Input: dimensioned drawing with shaded views. Units: mm. Origin: part minimum x, y, z. A direction names the side the tool comes from. Give positions to 0.01 mm unless a question says otherwise; leave off trailing zeros. Order: outer loops, then holes, each group sorted by start corner. A loop starts at its lowest first (then second) coordinate and runs counter-clockwise, first axis right, second up. Notation, with made-up numbers: (87, -7) -> (132, -7) arc R23 cw to (132, 30) -> close; hole circle Ø4 at (13, 62.5). An arc over 180 degrees is marked (long way). One line per question, with ' | ' between items. Start each with the question number.
(1) Section A-A (y = 41.5). Return loops of the section in (x, z), then the cut area to 3 significant figures.
(2) Section D-D (x = 6). Return loops of the section in (y, z).
(3) Set-up query: the marked faces 1 and 2. Return all of +Z, -Z, +X, -X, +Y, -Y with unobstructed straight access to the full face (end or side cutting, diameter ignored); none if empty.
(4) Section C-C (y = 20.5). Return loops of the section in (x, z) (1 decimal).
(5) First-contact query: pin 1 Ø4 at (x, y) = (39.23, 20.5) entering from -Z; pin 2 Ø1.5 at (x, z) = (30, 37) entering from +Y; pin 3 Ø1.5 at (x, y) = (44, 8) entering from -Z. Flat tips, straight axial feed; report the tip coordinate or a pass-through.
(6) Section B-B (x = 34). Return loops of the section in (y, z).
(7) Ray query, L1, parallel to X at y = 27, z = 51; L2, parallel to Z at x = 47, y = 42; L3, parallel to Y at x = 10, z = 3.5. Return the intervals inside material, ascending.
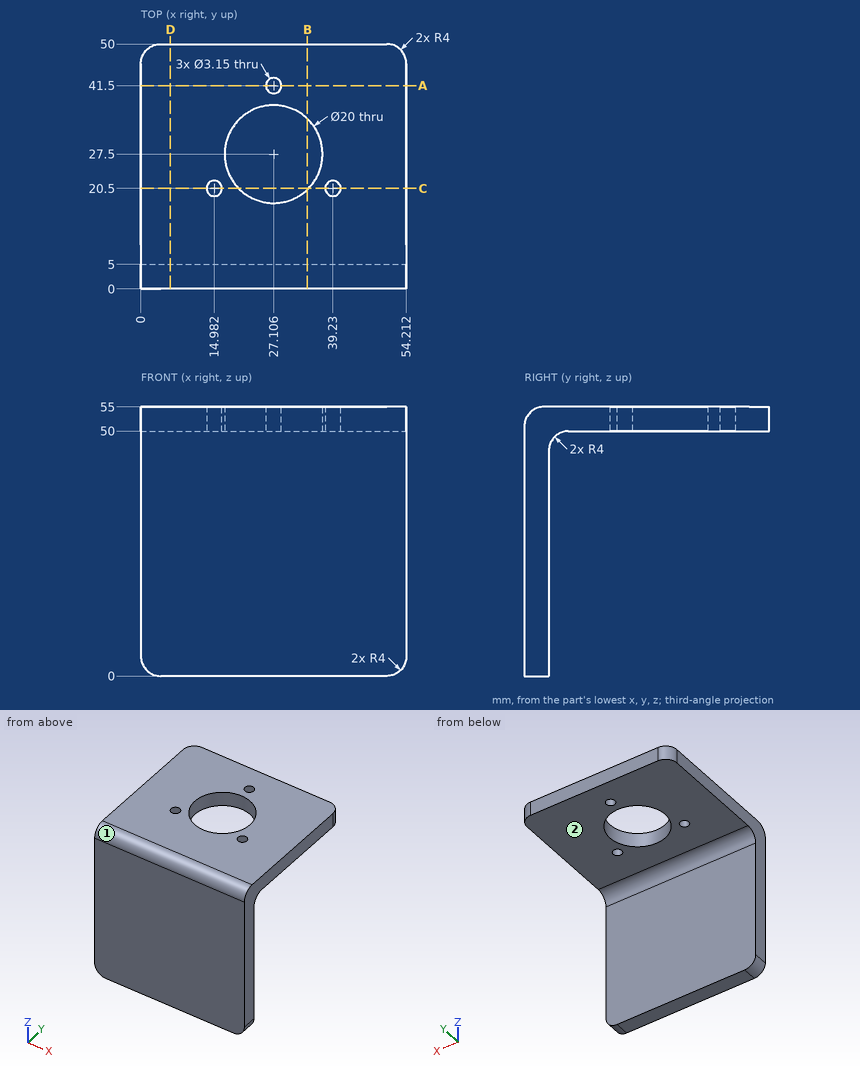
Response:
1) outline: (0, 50) -> (25.53, 50) -> (25.53, 55) -> (0, 55) -> close; (28.68, 50) -> (54.21, 50) -> (54.21, 55) -> (28.68, 55) -> close | area: 255 mm^2
2) outline: (0, 0) -> (5, 0) -> (5, 46) arc R4 cw to (9, 50) -> (50, 50) -> (50, 55) -> (4, 55) arc R4 ccw to (0, 51) -> close
3) face 1: +Z, +X, -X, -Y | face 2: -Z, +X, -X, +Y
4) outline: (0, 50) -> (13.4, 50) -> (13.4, 55) -> (0, 55) -> close; (16.6, 50) -> (20, 50) -> (20, 55) -> (16.6, 55) -> close; (34.2, 50) -> (37.7, 50) -> (37.7, 55) -> (34.2, 55) -> close; (40.8, 50) -> (54.2, 50) -> (54.2, 55) -> (40.8, 55) -> close
5) pin 1: stops at z = 50 | pin 2: stops at y = 5 | pin 3: stops at z = 49.6
6) outline: (0, 0) -> (5, 0) -> (5, 46) arc R4 cw to (9, 50) -> (20.26, 50) -> (20.26, 55) -> (4, 55) arc R4 ccw to (0, 51) -> close; (34.74, 50) -> (50, 50) -> (50, 55) -> (34.74, 55) -> close
7) L1: x = 0 to 17.12, 37.09 to 54.21 | L2: z = 50 to 55 | L3: y = 0 to 5
